```python
from build123d import *

# Parameters (mm, degrees)
F1_DEPTH       = 1549.4
F3_D           = 10.5664
F3_DEPTH       = 406.4
F3_CSINK_D     = 19.05
F3_CSINK_ANGLE = 82


with BuildPart() as f1:
    # F0 (on Right) → F1 (new body)
    with BuildSketch(Plane.YZ):
        with BuildLine():
            ThreePointArc((0, 3.175), (-13.09321, -2.037719), (-19.020937, -14.823125))
            Line((-19.020937, -14.823125), (-25.4, -130.175))
            Line((-25.4, -130.175), (-22.220149, -130.175))
            Line((-22.220149, -130.175), (-19.040298, -130.175))
            Line((-19.040298, -130.175), (-12.680625, -15.17375))
            ThreePointArc((-12.680625, -15.17375), (-8.728806, -6.650146), (0, -3.175))
            Line((0, -3.175), (304.8, -3.175))
            Line((304.8, -3.175), (304.8, 0))
            Line((304.8, 0), (304.8, 3.175))
            Line((304.8, 3.175), (0, 3.175))
        make_face()
    extrude(amount=F1_DEPTH)

    # F3
    with Locations(Plane.XY.offset(3.175)):
        with Locations((1530.35, 285.75), (1530.35, 19.05), (1225.55, 19.05), (1225.55, 285.75), (920.75, 285.75), (920.75, 19.05), (628.65, 285.75), (628.65, 19.05), (323.85, 19.05), (323.85, 285.75), (19.05, 285.75), (19.05, 19.05)):
            CounterSinkHole(F3_D / 2, F3_CSINK_D / 2, depth=F3_DEPTH, counter_sink_angle=F3_CSINK_ANGLE)


solid = f1.part
```
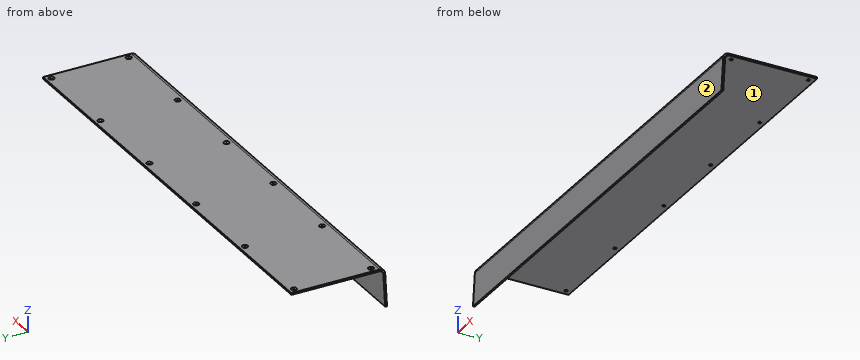
Check sheet for the modelled part. Datum: model origin and axes. Units: mm. Face numbers are marked on the shaded views. A direction names the side the tool comes from. Give positions to 0.01 mm unless a question says otherwise; leave off trailing zeros. Loops run counter-clockwise (first coordinate to the right, second up) from the corner with the lowest first, then second, coordinate; pieces in that order, holes last. Notation, with made-up numbers: M 48,62 L 80,62 A22 cw 80,85 Z; hole C 21,-25 d4. An arc over 180 degrees is marked long. Answer as CSV lines item,"result".
Item 1: Set-up check for the marked faces 1 and 2: record each of +Z, -Z, +X, -X, +Y, -Y from which the full face is reachable in a straight line by a thin tool's end or side.
Reply:
face 1,"-Z, +X, -X, +Y"
face 2,"+Z, +X, -X, -Y"
Item 2: Sectioned sample at A-A, the plane x = 761. Enter the section's corners in (y, z) (3 decimals), then the cut area to 3 significant figures.
Reply:
outline,"M -25.4,-130.175 L -19.04,-130.175 L -12.681,-15.174 A12.7 cw 0,-3.175 L 304.8,-3.175 L 304.8,3.175 L 0,3.175 A19.05 ccw -19.021,-14.823 Z"
area,"2,820 mm^2"
Item 3: Scan lines: L1, parallel to Y at x = 323, z = -2; L2, parallel to Y at x = 1530.35, z = -2.5; L3, parallel to Z at x = 308, y = 276 (3 decimals). Record each from-to range of solid material in increasing order.
Reply:
L1,"-13.05 to 13.84, 24.26 to 280.54, 290.96 to 304.8"
L2,"-13.57 to 13.77, 24.33 to 280.47, 291.03 to 304.8"
L3,"-3.175 to 3.175"
Item 4: Depth check by flat-ended pin: pin 1 Ø13.5 at (x, y) = (323.85, 19.05) entering from +Z; pin 2 Ø8 at (x, z) = (793, -89) entering from -Y; pin 3 Ø13.5 at (x, y) = (1530.35, 285.75) entering from -Z (3 decimals). Enter the tip coordinate at first touch or a pass-through.
Reply:
pin 1,"z = -0.02"
pin 2,"y = -23.34"
pin 3,"z = -3.175"
Item 5: Sectioned sample at C-C, the plane z = -100.5. Enter the section's corners in (x, y), then the cut area to 3 significant figures.
Reply:
outline,"M 0,-23.76 L 1549.4,-23.76 L 1549.4,-17.4 L 0,-17.4 Z"
area,"9,850 mm^2"
Item 6: Sectioned sample at B-B, the plane y = 167. Enter the section's corners in (x, z) (3 decimals), then the cut area to 3 significant figures.
Reply:
outline,"M 0,-3.175 L 1549.4,-3.175 L 1549.4,3.175 L 0,3.175 Z"
area,"9,840 mm^2"
